from build123d import *

# Parameters (mm, degrees)
BOSS_EXTRUDE3_DEPTH = 2
SKETCH6_W           = 10
SKETCH6_H           = 2
CUT_EXTRUDE4_DEPTH  = 2
CIRPATTERN3_COUNT   = 9
SKETCH7_R           = 7.5
CUT_EXTRUDE5_DEPTH  = 2


with BuildPart() as part:
    # Sketch1 → Boss-Extrude3 (new body)
    with BuildSketch(Plane(origin=(0, 0, 0), x_dir=(1, 0, 0), z_dir=(0, 1, 0))):
        with BuildLine():
            Line((-6.82662188, 21.439385106), (-4.862801047, 10.302003723))
            ThreePointArc((-4.862801047, 10.302003723), (-5.3476088, 9.262330141), (-6.49039641, 9.362311102))
            Line((-6.49039641, 9.362311102), (-15.153741203, 16.631720523))
            ThreePointArc((-15.153741203, 16.631720523), (-16.231142068, 15.582041817), (-17.23599997, 14.462721218))
            Line((-17.23599997, 14.462721218), (0, 0))
            Line((0, 0), (-22.5, 0))
            ThreePointArc((-22.5, 0), (-22.4497196, -1.503359534), (-22.299103121, -3))
            Line((-22.299103121, -3), (-10.989909678, -3))
            ThreePointArc((-10.989909678, -3), (-10.050217057, -3.657979857), (-10.347122068, -4.766044443))
            Line((-10.347122068, -4.766044443), (-19.010466861, -12.035453864))
            ThreePointArc((-19.010466861, -12.035453864), (-17.23599997, -14.462721218), (-15.153741203, -16.631720523))
            Line((-15.153741203, -16.631720523), (-6.49039641, -9.362311102))
            ThreePointArc((-6.49039641, -9.362311102), (-5.3476088, -9.262330141), (-4.862801047, -10.302003723))
            Line((-4.862801047, -10.302003723), (-6.82662188, -21.439385106))
            ThreePointArc((-6.82662188, -21.439385106), (-3.907083998, -22.158174443), (-0.917775362, -22.481274172))
            Line((-0.917775362, -22.481274172), (1.046045471, -11.343892789))
            ThreePointArc((1.046045471, -11.343892789), (1.857205046, -10.532733213), (2.896878628, -11.017540966))
            Line((2.896878628, -11.017540966), (8.551475349, -20.811589784))
            ThreePointArc((8.551475349, -20.811589784), (11.25, -19.485571585), (13.747627772, -17.811589784))
            Line((13.747627772, -17.811589784), (8.09303105, -8.017540966))
            ThreePointArc((8.09303105, -8.017540966), (8.193012011, -6.874753357), (9.301076597, -6.577848346))
            Line((9.301076597, -6.577848346), (19.928242223, -10.445820308))
            ThreePointArc((19.928242223, -10.445820308), (21.143083968, -7.695453225), (21.980363083, -4.807664583))
            Line((21.980363083, -4.807664583), (11.353197457, -0.939692621))
            ThreePointArc((11.353197457, -0.939692621), (10.695217601, 0), (11.353197457, 0.939692621))
            Line((11.353197457, 0.939692621), (21.980363083, 4.807664583))
            ThreePointArc((21.980363083, 4.807664583), (21.143083968, 7.695453225), (19.928242223, 10.445820308))
            Line((19.928242223, 10.445820308), (9.301076597, 6.577848346))
            ThreePointArc((9.301076597, 6.577848346), (8.193012011, 6.874753357), (8.09303105, 8.017540966))
            Line((8.09303105, 8.017540966), (13.747627772, 17.811589784))
            ThreePointArc((13.747627772, 17.811589784), (11.25, 19.485571585), (8.551475349, 20.811589784))
            Line((8.551475349, 20.811589784), (2.896878628, 11.017540966))
            ThreePointArc((2.896878628, 11.017540966), (1.857205046, 10.532733213), (1.046045471, 11.343892789))
            Line((1.046045471, 11.343892789), (-0.917775362, 22.481274172))
            ThreePointArc((-0.917775362, 22.481274172), (-3.907083998, 22.158174443), (-6.82662188, 21.439385106))
        make_face()
        with BuildLine():
            Line((0, 0), (-17.23599997, 14.462721218))
            ThreePointArc((-17.23599997, 14.462721218), (-18.163823831, 13.278761383), (-19.010466861, 12.035453864))
            Line((-19.010466861, 12.035453864), (-10.347122068, 4.766044443))
            ThreePointArc((-10.347122068, 4.766044443), (-10.050217057, 3.657979857), (-10.989909678, 3))
            Line((-10.989909678, 3), (-22.299103121, 3))
            ThreePointArc((-22.299103121, 3), (-22.4497196, 1.503359534), (-22.5, 0))
            Line((-22.5, 0), (0, 0))
        make_face()
    extrude(amount=BOSS_EXTRUDE3_DEPTH)

    # Sketch6 → Cut-Extrude4 (cut)
    with BuildSketch(Plane(origin=(0, 2, 0), x_dir=(1, 0, 0), z_dir=(0, 1, 0))):
        with Locations((-22.5, 0)):
            Rectangle(SKETCH6_W, SKETCH6_H)
    cut_extrude4 = extrude(amount=-CUT_EXTRUDE4_DEPTH, mode=Mode.SUBTRACT)

    # CirPattern3: Cut-Extrude4 ×9 about axis
    cirpattern3_axis = Axis((0, 0, 0), (0, 1, 0))
    for i in range(1, CIRPATTERN3_COUNT):
        add(cut_extrude4.rotate(cirpattern3_axis, i * 360 / CIRPATTERN3_COUNT), mode=Mode.SUBTRACT)

    # Sketch7 → Cut-Extrude5 (cut)
    with BuildSketch(Plane(origin=(0, 2, 0), x_dir=(1, 0, 0), z_dir=(0, 1, 0))):
        with Locations(Location((0, 0, 0), (0, 0, 270))):
            Circle(SKETCH7_R)
    extrude(amount=-CUT_EXTRUDE5_DEPTH, mode=Mode.SUBTRACT)


solid = part.part
Could you check a few things on this model? Use its own coordinates, in mm. A direction names the side the tool comes from. Give positions to 0.01 mm unless a question says otherwise; leave off trailing zeros. Order: outer loops, then holes, each group sorted by start corner. A loop starts at its lowest first (then second) coordinate and runs counter-clockwise, first axis right, second up. Notation, with made-up numbers: (24, 86) - (68, 86) arc R35 ccw to (68, 121) - close; hole circle Ø6 at (58.25, 29). An arc over 180 degrees is marked (long way). Return JSON: item names as keys, results as strings. Group by question number.
Q1. Suppose I cut it at C-C, the plane x = 17.5. Please give me the cut outline in (y, z).
Q2. Which directions (+Z, -Z, +X, -X, +Y, -Y) give clear straight access to the entire face, cutting with the end or side of a thin tool? Please do faces 4 (the face through (16.45, 1.01, 5.97)), 5 (the face through (0.08, 0.99, -16.83)), 6 (the face through (5.685, 0.986, 15.846)).
Q3. Suppose I cut it at A-A, the plane z = 0. Please give me the cut outline in (x, y), and give its area (3 significant figures).
Q4. Suppose I cut it at B-B, the plane z = -13. Please give me the cut outline in (x, y).
Q5. Will these pins go through, and if not, where does the flat tip stop? pin 1 Ø8 at (x, z) = (3, 13) entering from -Y; pin 2 Ø1 at (y, z) = (1, 17) entering from +X; pin 3 Ø0.6 at (y, z) = (1.5, 0.5) entering from -X; pin 4 Ø1 at (y, z) = (1.5, -12) entering from -X.
Q6. Please list where these lines run through material, in increasing order: line 1 along X through (y, z) = (0.8, 0); line 2 along Z through (x, y) = (-19.5, 1.2); line 3 along X through (y, z) = (1, 18). Write a range as [from, to].
Q7. Thinking about a two-plate mould opening in X: for faces 1 (the face through (-18.45, 0.99, -12.88)), 2 (the face through (9.484, 0.986, -20.403)), 3 (the face through (8.204, 0.986, -6.862)), which applies, pulls with the +X half, pulls with the -X half, needs draft (parallel to the pull), parting line crosses it, or undercut?
Q8. Suppose I cut it at D-D, the plane x = 0. Please give me the cut outline in (y, z), and give its area (3 significant figures).
Resolved:
{
 "1": {"outline": "(0, -9.56) - (2, -9.56) - (2, -7.43) - (0, -7.43) - close; (0, -5.31) - (2, -5.31) - (2, -3.18) - (0, -3.18) - close; (0, 3.18) - (2, 3.18) - (2, 5.31) - (0, 5.31) - close; (0, 7.43) - (2, 7.43) - (2, 9.56) - (0, 9.56) - close"},
 "2": {"face 4": "+Y, -Y", "face 5": "-Z, +Y, -Y", "face 6": "+Z, +Y, -Y"},
 "3": {"outline": "(-17.5, 0) - (-7.5, 0) - (-7.5, 2) - (-17.5, 2) - close; (7.5, 0) - (10.7, 0) - (10.7, 2) - (7.5, 2) - close", "area": "26.4 mm2"},
 "4": {"outline": "(-18.36, 0) - (-17.05, 0) - (-17.05, 2) - (-18.36, 2) - close; (-13.94, 0) - (-10.83, 0) - (-10.83, 2) - (-13.94, 2) - close; (-5.34, 0) - (0.75, 0) - (0.75, 2) - (-5.34, 2) - close; (4.04, 0) - (10.97, 0) - (10.97, 2) - (4.04, 2) - close"},
 "5": {"pin 1": "stops at y = 0", "pin 2": "stops at x = 13.57", "pin 3": "stops at x = -17.5", "pin 4": "stops at x = -19.01"},
 "6": {"line 1": "x = [-17.5, -7.5], [7.5, 10.7]", "line 2": "z = [-3, -1], [1, 3]", "line 3": "x = [-6.22, -4.19], [-2.16, -0.13], [6.93, 9.24], [11.55, 13.5]"},
 "7": {"face 1": "pulls with the -X half", "face 2": "pulls with the +X half", "face 3": "undercut"},
 "8": {"outline": "(0, -17.28) - (2, -17.28) - (2, -7.5) - (0, -7.5) - close; (0, 7.5) - (2, 7.5) - (2, 17.28) - (0, 17.28) - close", "area": "39.1 mm2"}
}
